```python
from build123d import *

# Parameters (mm, degrees)
SKETCH_1_W          = 78
SKETCH_1_H          = 78
SKETCH_1_R          = 23.75
EXTRUDE_1_DEPTH     = 2
EXTRUDE_START       = 4
SKETCH_2_R          = 30.9
SKETCH_2_R_2        = 23.75
EXTRUDE_2_DEPTH     = 4
SKETCH_3_W          = 78
SKETCH_3_H          = 78
SKETCH_3_W_2        = 74
SKETCH_3_H_2        = 74
SKETCH_3_W_3        = 5
SKETCH_3_H_3        = 5
EXTRUDE_3_DEPTH     = 4
SKETCH_4_R          = 0.75
CUT_EXTRUDE_1_DEPTH = 5
CUT_EXTRUDE_2_DEPTH = 4
SKETCH_6_R          = 1.05
SKETCH_6_R_2        = 0.55
EXTRUDE_4_DEPTH     = 2
EXTRUDE_START_2     = 1.5
EXTRUDE_5_DEPTH     = 1.5
CHAMFER_1_SIZE      = 0.5
SKETCH_9_R          = 1.65
SKETCH_9_R_2        = 0.8
EXTRUDE_6_DEPTH     = 2
CUT_EXTRUDE_START   = -2
SKETCH_9_2_R        = 0.8
CUT_EXTRUDE_4_DEPTH = 2
SKETCH_10_R         = 0.8
CUT_EXTRUDE_5_DEPTH = 4
FILLET_2_R          = 1.5
FILLET_3_R          = 3.5
CHAMFER_2_SIZE      = 1
SKETCH_11_R         = 24.25
CUT_EXTRUDE_6_DEPTH = 1
SKETCH_12_W         = 50
SKETCH_12_H         = 1
SKETCH_12_W_2       = 1
SKETCH_12_H_2       = 50
CUT_EXTRUDE_7_DEPTH = 1
EXTRUDE_START_3     = -3
SKETCH_14_R         = 0.8
EXTRUDE_7_DEPTH     = 3


with BuildPart() as part:
    # Sketch 1 → Extrude 1 (new body)
    with BuildSketch(Plane.XY):
        Rectangle(SKETCH_1_W, SKETCH_1_H)
        Circle(SKETCH_1_R, mode=Mode.SUBTRACT)
    extrude(amount=-EXTRUDE_1_DEPTH)

    # Sketch 2 → Extrude 2 (add)
    with BuildSketch(Plane.XY.offset(EXTRUDE_START)):
        with Locations(Location((0, 0, 0), (0, 0, 180))):
            Circle(SKETCH_2_R)
        Circle(SKETCH_2_R_2, mode=Mode.SUBTRACT)
    extrude(amount=-EXTRUDE_2_DEPTH)

    # Sketch 3 → Extrude 3 (add)
    # profile 1 of 5: a face of its own
    with BuildSketch(Plane(origin=(0, 0, -2), x_dir=(-1, 0, 0), z_dir=(0, 0, -1))):
        Rectangle(SKETCH_3_W, SKETCH_3_H)
        Rectangle(SKETCH_3_W_2, SKETCH_3_H_2, mode=Mode.SUBTRACT)
    # profile 2 of 5: a face of its own
    with BuildSketch(Plane(origin=(0, 0, -2), x_dir=(-1, 0, 0), z_dir=(0, 0, -1))):
        with Locations((-34.5, 34.5)):
            Rectangle(SKETCH_3_W_3, SKETCH_3_H_3)
    # profile 3 of 5: a face of its own
    with BuildSketch(Plane(origin=(0, 0, -2), x_dir=(-1, 0, 0), z_dir=(0, 0, -1))):
        with Locations((34.5, 34.5)):
            Rectangle(SKETCH_3_W_3, SKETCH_3_H_3)
    # profile 4 of 5: a face of its own
    with BuildSketch(Plane(origin=(0, 0, -2), x_dir=(-1, 0, 0), z_dir=(0, 0, -1))):
        with Locations((34.5, -34.5)):
            Rectangle(SKETCH_3_W_3, SKETCH_3_H_3)
    # profile 5 of 5: a face of its own
    with BuildSketch(Plane(origin=(0, 0, -2), x_dir=(-1, 0, 0), z_dir=(0, 0, -1))):
        with Locations((-34.5, -34.5)):
            Rectangle(SKETCH_3_W_3, SKETCH_3_H_3)
    extrude(amount=EXTRUDE_3_DEPTH)

    # Sketch 4 → Cut-Extrude 1 (cut)
    with BuildSketch(Plane.XY.offset(4)):
        with Locations((0, 26)):
            Circle(SKETCH_4_R)
        with Locations((26, 0)):
            Circle(SKETCH_4_R)
        with Locations((0, -26)):
            Circle(SKETCH_4_R)
        with Locations((-26, 0)):
            Circle(SKETCH_4_R)
    extrude(amount=-CUT_EXTRUDE_1_DEPTH, mode=Mode.SUBTRACT)

    # Sketch 5 → Cut-Extrude 2 (cut)
    with BuildSketch(Plane.XY.offset(4)):
        with BuildLine():
            Line((-27.974819843, -13.719309558), (-23.559323961, -20.390396134))
            Line((-23.559323961, -20.390396134), (-22.644398758, -19.59853609))
            Line((-22.644398758, -19.59853609), (-23.332248508, -18.55930848))
            Line((-23.332248508, -18.55930848), (-20.696942595, -16.463091505))
            ThreePointArc((-20.696942595, -16.463091505), (-19.966595187, -15.210744122), (-20.274200224, -13.794001221))
            Line((-20.274200224, -13.794001221), (-20.619206205, -13.272754043))
            ThreePointArc((-20.619206205, -13.272754043), (-21.803134058, -12.436036561), (-23.24129537, -12.618993788))
            Line((-23.24129537, -12.618993788), (-26.200569323, -14.225748447))
            Line((-26.200569323, -14.225748447), (-26.888419073, -13.186520837))
            Line((-26.888419073, -13.186520837), (-27.974819843, -13.719309558))
        make_face()
    extrude(amount=-CUT_EXTRUDE_2_DEPTH, mode=Mode.SUBTRACT)

    # Sketch 6 → Extrude 4 (add)
    with BuildSketch(Plane.XY):
        with Locations(Location((-22.409013696, -14.832202606, 0), (0, 0, 180))):
            Circle(SKETCH_6_R)
        with Locations((-22.409013696, -14.832202606)):
            Circle(SKETCH_6_R_2, mode=Mode.SUBTRACT)
    extrude(amount=EXTRUDE_4_DEPTH)

    # Sketch 8 → Extrude 5 (add)
    with BuildSketch(Plane.XY.offset(4).offset(EXTRUDE_START_2)):
        with BuildLine():
            ThreePointArc((30.9, 0), (-6.983586682, 30.100490312), (-27.743334437, -13.605785326))
            Line((-27.743334437, -13.605785326), (-26.888419073, -13.186520837))
            Line((-26.888419073, -13.186520837), (-26.329232439, -12.912286559))
            ThreePointArc((-26.329232439, -12.912286559), (-6.627627167, 28.56624202), (29.325, 0))
            ThreePointArc((29.325, 0), (10.240081174, -27.479016768), (-22.17347315, -19.190953949))
            Line((-22.17347315, -19.190953949), (-22.644398758, -19.59853609))
            Line((-22.644398758, -19.59853609), (-23.3643758, -20.221670146))
            ThreePointArc((-23.3643758, -20.221670146), (10.790059958, -28.954871889), (30.9, 0))
        make_face()
    extrude(amount=-EXTRUDE_5_DEPTH)

    # Chamfer 1
    chamfer_1_edges = [part.edges().sort_by_distance(p)[0] for p in [
        (25.767071902, 17.054852846, 5.5),
    ]]
    chamfer(chamfer_1_edges, length=CHAMFER_1_SIZE)

    # Sketch 9 → Extrude 6 (add)
    # profile 1 of 3: a face of its own
    with BuildSketch(Plane(origin=(0, 0, -2), x_dir=(-1, 0, 0), z_dir=(0, 0, -1))):
        with Locations((-19, -19)):
            Circle(SKETCH_9_R)
        with Locations((-19, -19)):
            Circle(SKETCH_9_R_2, mode=Mode.SUBTRACT)
    # profile 2 of 3: a face of its own
    with BuildSketch(Plane(origin=(0, 0, -2), x_dir=(-1, 0, 0), z_dir=(0, 0, -1))):
        with Locations((-19, 19)):
            Circle(SKETCH_9_R)
        with Locations((-19, 19)):
            Circle(SKETCH_9_R_2, mode=Mode.SUBTRACT)
    # profile 3 of 3: a face of its own
    with BuildSketch(Plane(origin=(0, 0, -2), x_dir=(-1, 0, 0), z_dir=(0, 0, -1))):
        with Locations((19, 19)):
            Circle(SKETCH_9_R)
        with Locations((19, 19)):
            Circle(SKETCH_9_R_2, mode=Mode.SUBTRACT)
    extrude(amount=EXTRUDE_6_DEPTH)

    # Sketch 9_2 → Cut-Extrude 4 (cut)
    with BuildSketch(Plane(origin=(0, 0, -2), x_dir=(-1, 0, 0), z_dir=(0, 0, -1)).offset(CUT_EXTRUDE_START)):
        with Locations((-19, 19)):
            Circle(SKETCH_9_2_R)
        with Locations((19, 19)):
            Circle(SKETCH_9_2_R)
        with Locations((-19, -19)):
            Circle(SKETCH_9_2_R)
    extrude(amount=CUT_EXTRUDE_4_DEPTH, mode=Mode.SUBTRACT)

    # Sketch 10 → Cut-Extrude 5 (cut)
    with BuildSketch(Plane(origin=(0, 0, -6), x_dir=(-1, 0, 0), z_dir=(0, 0, -1))):
        with Locations((-34.5, 34.5)):
            Circle(SKETCH_10_R)
        with Locations((34.5, 34.5)):
            Circle(SKETCH_10_R)
        with Locations((34.5, -34.5)):
            Circle(SKETCH_10_R)
        with Locations((-34.5, -34.5)):
            Circle(SKETCH_10_R)
    extrude(amount=-CUT_EXTRUDE_5_DEPTH, mode=Mode.SUBTRACT)

    # Fillet 2
    fillet_2_edges = [part.edges().sort_by_distance(p)[0] for p in [
        (-37, 32, -4),
        (-37, -32, -4),
        (-32, -32, -4),
        (-32, -37, -4),
        (32, -37, -4),
        (32, -32, -4),
        (37, -32, -4),
        (37, 32, -4),
        (32, 32, -4),
        (32, 37, -4),
        (-32, 37, -4),
        (-32, 32, -4),
    ]]
    fillet(fillet_2_edges, radius=FILLET_2_R)

    # Fillet 3
    fillet_3_edges = [part.edges().sort_by_distance(p)[0] for p in [
        (39, -39, -3),
        (-39, -39, -3),
        (-39, 39, -3),
        (39, 39, -3),
    ]]
    fillet(fillet_3_edges, radius=FILLET_3_R)

    # Chamfer 2
    chamfer_2_edges = [part.edges().sort_by_distance(p)[0] for p in [
        (0, -39, 0),
        (39, 0, 0),
        (0, 39, 0),
        (-39, 0, 0),
        (37.974873734, 37.974873734, 0),
        (-37.974873734, 37.974873734, 0),
        (-37.974873734, -37.974873734, 0),
        (37.974873734, -37.974873734, 0),
    ]]
    chamfer(chamfer_2_edges, length=CHAMFER_2_SIZE)

    # Sketch 11 → Cut-Extrude 6 (cut)
    with BuildSketch(Plane.XY.offset(4)):
        Circle(SKETCH_11_R)
    extrude(amount=-CUT_EXTRUDE_6_DEPTH, mode=Mode.SUBTRACT)

    # Sketch 12 → Cut-Extrude 7 (cut)
    with BuildSketch(Plane(origin=(0, 0, -6), x_dir=(-1, 0, 0), z_dir=(0, 0, -1))):
        with Locations((0, 37.5)):
            Rectangle(SKETCH_12_W, SKETCH_12_H)
        with Locations((37.5, 0)):
            Rectangle(SKETCH_12_W_2, SKETCH_12_H_2)
        with Locations((0, -37.5)):
            Rectangle(SKETCH_12_W, SKETCH_12_H)
        with Locations((-37.5, 0)):
            Rectangle(SKETCH_12_W_2, SKETCH_12_H_2)
    extrude(amount=-CUT_EXTRUDE_7_DEPTH, mode=Mode.SUBTRACT)

    # Sketch 14 → Extrude 7 (add)
    with BuildSketch(Plane(origin=(0, 0, -2), x_dir=(-1, 0, 0), z_dir=(0, 0, -1)).offset(EXTRUDE_START_3)):
        with BuildLine():
            Line((-12.128891128, -13.3), (-19.676699418, -13.3))
            ThreePointArc((-19.676699418, -13.3), (0, -23.75), (19.676699418, -13.3))
            Line((19.676699418, -13.3), (12.128891128, -13.3))
            ThreePointArc((12.128891128, -13.3), (11.999124031, -13.417191304), (11.868224672, -13.533116535))
            ThreePointArc((11.868224672, -13.533116535), (-0.174850165, -17.999150742), (-12.128891128, -13.3))
        make_face()
        with Locations((-3.804261279, -19.125312968)):
            Circle(SKETCH_14_R, mode=Mode.SUBTRACT)
        with Locations((-1.27536102, -19.458249003)):
            Circle(SKETCH_14_R, mode=Mode.SUBTRACT)
        with Locations((-8.624629459, -17.48901846)):
            Circle(SKETCH_14_R, mode=Mode.SUBTRACT)
        with Locations((-6.268069573, -18.465137525)):
            Circle(SKETCH_14_R, mode=Mode.SUBTRACT)
        with Locations((1.27536102, -19.458249003)):
            Circle(SKETCH_14_R, mode=Mode.SUBTRACT)
        with Locations((3.804261279, -19.125312968)):
            Circle(SKETCH_14_R, mode=Mode.SUBTRACT)
        with Locations((6.268069573, -18.465137525)):
            Circle(SKETCH_14_R, mode=Mode.SUBTRACT)
        with Locations((8.624629459, -17.48901846)):
            Circle(SKETCH_14_R, mode=Mode.SUBTRACT)
        with Locations((10.833619544, -16.21365744)):
            Circle(SKETCH_14_R, mode=Mode.SUBTRACT)
        with BuildLine():
            ThreePointArc((13.657243394, -14.660876246), (12.527077771, -15.389567306), (12.329766742, -14.0594044))
            ThreePointArc((12.329766742, -14.0594044), (13.187409018, -13.932185186), (13.657243394, -14.660876246))
        make_face(mode=Mode.SUBTRACT)
    extrude(amount=EXTRUDE_7_DEPTH)


solid = part.part
```
Geometry check sheet. Reference: the model listing, model coordinates, mm. A direction names the side the tool comes from. Give positions to 0.01 mm unless a question says otherwise; leave off trailing zeros. Use one line per item in the form item = value.
Item 1: Mould release check, pull along X, two halves, no side actions. Record for faces 4 (the flat face through (-39, 0, -3)), 5 (the flat face through (-37, 0, -4)), 6 (the cylindrical face through (20.216, 20.115, -2.986)), 7 (the cylindrical face through (38, -37.95, -3.54)): released by +X, released by -X, zero draft, split by the parting line, or undercut.
Results list:
face_4 = released by -X
face_5 = undercut
face_6 = undercut
face_7 = released by +X
Item 2: Sectioned sample at A-A on z = -3. Count the separate pieces of the cut face and the enclosed holes in it, plus the area to 3 significant figures.
Results list:
separate_pieces = 4
enclosed_holes = 8
area = 711 mm2
Item 3: Access from +Z, -Z, +X, -X, +Y, -Y to the whole of each face (thin tool, end or side, straight path). Record for faces 1 (the conical face through (-37.5, 37.6, -0.4)), 2 (the cylindrical face through (-18.785, 20.636, -2.986)), 3 (the cylindrical face through (26.463, 15.953, 2.535)).
Results list:
face_1 = +Z, -X, +Y
face_2 = -Z
face_3 = +Z
Item 4: Scan lines: line 1 (Y direction, x = -19, z = -2.75); line 2 (Y direction, x = -34.5, z = -4.7); line 3 (Y direction, x = 11.5, z = -3.75). Record each from-to range of solid material in increasing order.
Results list:
line_1 = -39 to -37, 17.35 to 18.2, 19.8 to 20.65, 37 to 39
line_2 = -39 to -35.3, -33.7 to -32, 32 to 33.7, 35.3 to 39
line_3 = -39 to -37, 37 to 39
Item 5: Depth check by flat-ended pin: pin 1 Ø1.8 at (x, y) = (8.62, -17.49) entering from +Z; pin 2 Ø2.5 at (x, y) = (3.8, -19.13) entering from -Z; pin 3 Ø2 at (x, y) = (-34.5, -34.5) entering from +Z. Enter the tip coordinate at first touch or a pass-through.
Results list:
pin_1 = 1
pin_2 = -2
pin_3 = 0
